Can you work these out from the model? Positions are in its coordinate system, mm. A direction names the side the tool comes from. Coordinates: 2 decimals unless noted, no trailing zeros. Write each loop counter-clockwise with the first axis right and the second up, starting at its lowest first coordinate (ties: lowest second). Pieces come first, ordered by that corner, then holes. Notation, with made-up numbers: (-32, -18) -> (-26, -18) arc R19 ccw to (-26, -10) -> close; hole circle Ø11 at (-7.5, -37.5). An arc over 180 degrees is marked (long way). Use one line per item in the form item = value.
```python
from build123d import *

# Parameters (mm, degrees)
SKETCH_1_R      = 1.55
EXTRUDE_1_DEPTH = 2


with BuildPart() as part:
    # 草图1 → 凸台-拉伸1 (new body)
    with BuildSketch(Plane.XY):
        with BuildLine():
            Line((-4.5, 10), (4.5, 10))
            Line((4.5, 10), (42.874156462, 10))
            ThreePointArc((42.874156462, 10), (44.288370024, 9.414213562), (44.874156462, 8))
            Line((44.874156462, 8), (44.874156462, 5.149651674))
            ThreePointArc((44.874156462, 5.149651674), (44.458733517, 3.929358448), (43.385040906, 3.216003028))
            Line((43.385040906, 3.216003028), (31.212777732, 0))
            Line((31.212777732, 0), (4.5, -7))
            Line((4.5, -7), (-4.5, -7))
            Line((-4.5, -7), (-4.5, 10))
        make_face()
        with Locations((-0.5, 6.5)):
            Circle(SKETCH_1_R, mode=Mode.SUBTRACT)
        with Locations((40.890589187, 6.411336053)):
            Circle(SKETCH_1_R, mode=Mode.SUBTRACT)
        with Locations((-0.5, -3.5)):
            Circle(SKETCH_1_R, mode=Mode.SUBTRACT)
        with BuildLine():
            Line((4.146506743, 5.745070559), (4.146506743, -3.06967977))
            ThreePointArc((4.146506743, -3.06967977), (4.535559953, -3.861351432), (5.399994782, -4.037018291))
            Line((5.399994782, -4.037018291), (12.9777079, -2.051302228))
            ThreePointArc((12.9777079, -2.051302228), (13.695890464, -1.320302954), (13.3936769, -0.341112934))
            Line((13.3936769, -0.341112934), (5.815963783, 6.487921333))
            ThreePointArc((5.815963783, 6.487921333), (4.739970791, 6.658705344), (4.146506743, 5.745070559))
        make_face(mode=Mode.SUBTRACT)
        with BuildLine():
            Line((11.315621432, 5.017151032), (17.427365311, -0.490751911))
            ThreePointArc((17.427365311, -0.490751911), (17.860483104, -0.71957174), (18.35031039, -0.715239658))
            Line((18.35031039, -0.715239658), (24.045702218, 0.777219988))
            ThreePointArc((24.045702218, 0.777219988), (24.791574656, 1.708800456), (24.11419002, 2.691306394))
            Line((24.11419002, 2.691306394), (12.307054312, 6.706749691))
            ThreePointArc((12.307054312, 6.706749691), (11.122598499, 6.266093001), (11.315621432, 5.017151032))
        make_face(mode=Mode.SUBTRACT)
        with BuildLine():
            Line((20.321587877, 5.773595304), (31.417514437, 2.000024386))
            ThreePointArc((31.417514437, 2.000024386), (32.013649619, 1.98508799), (32.512293671, 2.312126767))
            Line((32.512293671, 2.312126767), (35.611244636, 6.085697684))
            ThreePointArc((35.611244636, 6.085697684), (35.742500286, 7.147750779), (34.838441243, 7.720343189))
            Line((34.838441243, 7.720343189), (20.643563718, 7.720343189))
            ThreePointArc((20.643563718, 7.720343189), (19.656966565, 6.883518118), (20.321587877, 5.773595304))
        make_face(mode=Mode.SUBTRACT)
    extrude(amount=EXTRUDE_1_DEPTH)


solid = part.part
```
Q1. Thinking about a two-plate mould opening in X: for faces 1 (the flat face through (0, -7, 1)), 2 (the cylindrical face through (17.854, -0.718, 0.986)), 3 (the flat face through (37.38, 1.63, 0.99)), which applies, released by +X, released by -X, zero draft, split by the parting line, or undercut?
Return value:
face_1 = zero draft
face_2 = undercut
face_3 = released by +X
Q2. Suppose I cut it at B-B (y = -4.5). Write out the boundary of the cut face in (x, z).
Return value:
outline = (-4.5, 0) -> (-1.68, 0) -> (-1.68, 2) -> (-4.5, 2) -> close; (0.68, 0) -> (14.04, 0) -> (14.04, 2) -> (0.68, 2) -> close
Q3. Will these pins go through, and if not, where does the flat tip stop? pin 1 (1.9 mm diameter, centred on x = 40.89, y = 6.41, fed in from +Z); pin 2 (0.6 mm diameter, centred on y = 3.5, z = 1, fed in from +X); pin 3 (1 mm diameter, centred on x = 27, z = 1.5, fed in from -Y).
Return value:
pin_1 = through
pin_2 = 44.35
pin_3 = -1.23
Q4. For faces 4 (the flat face through (19, 10, 1)), 5 (the flat face through (4.147, 1, 1)), which set-ups out of +Z, -Z, +X, -X, +Y, -Y let a thin tool reach every point of the face, with its end or its side?
Return value:
face_4 = +Z, -Z, +X, -X, +Y
face_5 = +Z, -Z
Q5. If I drill on line 1 (Y direction, x = -0.5, z = 1); line 2 (Y direction, x = 20.5, z = 0.6); line 3 (Y direction, x = 6, z = 1.05), over which ranges is the centre line in solid material (lowest first)? Write a range as from..to.
Return value:
line_1 = -7..-5.05, -1.95..4.95, 8.05..10
line_2 = -2.81..-0.15, 3.92..5.71, 7.71..10
line_3 = -6.61..-3.88, 6.32..10
Q6. Suppose I cut it at D-D (y = 4). Write out the boundary of the cut face in (x, z), then the cut area to 3 significant figures.
Return value:
outline = (-4.5, 0) -> (4.15, 0) -> (4.15, 2) -> (-4.5, 2) -> close; (8.58, 0) -> (12.44, 0) -> (12.44, 2) -> (8.58, 2) -> close; (20.27, 0) -> (25.54, 0) -> (25.54, 2) -> (20.27, 2) -> close; (33.9, 0) -> (44.51, 0) -> (44.51, 2) -> (33.9, 2) -> close
area = 56.8 mm2
Q7. Suppose I cut it at A-A (x = -0.5). Write out the boundary of the cut face in (y, z), then the cut area to 3 significant figures.
Return value:
outline = (-7, 0) -> (-5.05, 0) -> (-5.05, 2) -> (-7, 2) -> close; (-1.95, 0) -> (4.95, 0) -> (4.95, 2) -> (-1.95, 2) -> close; (8.05, 0) -> (10, 0) -> (10, 2) -> (8.05, 2) -> close
area = 21.6 mm2
Q8. Suppose I cut it at C-C (x = 17). Write out the boundary of the cut face in (y, z), then the cut area to 3 significant figures.
Return value:
outline = (-3.72, 0) -> (-0.11, 0) -> (-0.11, 2) -> (-3.72, 2) -> close; (5.11, 0) -> (10, 0) -> (10, 2) -> (5.11, 2) -> close
area = 17.0 mm2
